from build123d import *

# Parameters (mm, degrees)
BASE_FLANGE1_DEPTH      = 300
CUT_EXTRUDE1_DEPTH      = 303.226736077
CUT_EXTRUDE1_DEPTH_BACK = 303.226736077
SKETCH7_R               = 3


# Sheet-metal steps are written as plain solids
with BuildPart() as part:
    # Sketch2 → Base-Flange1 (new body)
    with BuildSketch(Plane(origin=(0, 0, 0), x_dir=(0, 0, -1), z_dir=(1, 0, 0))):
        with BuildLine():
            Line((0, 0), (18, 0))
            ThreePointArc((18, 0), (19.414213562, -0.585786438), (20, -2))
            Line((20, -2), (20, -19))
            ThreePointArc((20, -19), (20.292893219, -19.707106781), (21, -20))
            Line((21, -20), (30, -20))
            Line((30, -20), (30, -21))
            Line((30, -21), (21, -21))
            ThreePointArc((21, -21), (19.585786438, -20.414213562), (19, -19))
            Line((19, -19), (19, -2))
            ThreePointArc((19, -2), (18.707106781, -1.292893219), (18, -1))
            Line((18, -1), (0, -1))
            Line((0, -1), (0, 0))
        make_face()
    extrude(amount=BASE_FLANGE1_DEPTH)

    # Sketch7 → Cut-Extrude1 (cut, two sides: drawn at the far end of the back side and taken through both)
    with BuildSketch(Plane(origin=(0, 0, 0), x_dir=(1, 0, 0), z_dir=(0, 1, 0)).offset(-CUT_EXTRUDE1_DEPTH_BACK)):
        with Locations(Location((50, 9, 0), (0, 0, 270))):
            Circle(SKETCH7_R)
        with Locations(Location((150, 9, 0), (0, 0, 270))):
            Circle(SKETCH7_R)
    extrude(amount=CUT_EXTRUDE1_DEPTH + CUT_EXTRUDE1_DEPTH_BACK, mode=Mode.SUBTRACT)


solid = part.part
Here's how the part is built. I have some questions about the finished solid (model axes, mm). A direction names the side the tool comes from. Give positions to 0.01 mm unless a question says otherwise; leave off trailing zeros. Write each loop counter-clockwise with the first axis right and the second up, starting at its lowest first coordinate (ties: lowest second). Pieces come first, ordered by that corner, then holes. Notation, with made-up numbers: (63.25, -6) -> (101.25, -6) arc R21 cw to (101.25, 30) -> close; hole circle Ø8 at (-2, 43). An arc over 180 degrees is marked (long way). Use one line per item in the form item = value. Start each with the question number.
1. On a 3-axis mill with a long thin cutter (end or side, diameter ignored), from which of +Z, -Z, +X, -X, +Y, -Y can I reach the whole of each face in a straight line? I mean faces 1 (the face through (0, -8.9, -19.5)), 2 (the face through (148, -1, -5)), 3 (the face through (148, -10, -20)). Say none if no direction works.
2. Will these pins go through, and if not, where does the flat tip stop? pin 1 Ø12 at (x, y) = (94.5, -18) entering from +Z; pin 2 Ø7 at (x, z) = (117.5, -26) entering from +Y; pin 3 Ø2 at (x, y) = (136, -18.5) entering from -Z.
3. Thinking about a two-plate mould opening in X: for faces 4 (the face through (152.53, -0.51, -7.39)), 5 (the face through (52.974, -0.507, -9.391)), 6 (the face through (148, -20, -25)), 7 (the face through (300, -8.9, -19.5)), which applies, +X half, -X half, draft (parallel to the pull), parting line (faces both ways), or undercut?
4. Imagine slicing it at A-A on z = -9. List the corners of the cut face in (x, y) for me.
5. If I drill on L1, parallel to X at y = -0.35, z = -9; L2, parallel to Z at x = 221.5, y = -7.5; L3, parallel to Y at x = 255, z = -22.5, over which ranges is the centre line in solid material (lowest first)?
6. Imagine slicing it at C-C on x = 150. List the corners of the cut face in (y, z) for me.
7. Imagine slicing it at B-B on x = 202. List the corners of the cut face in (y, z) for me, plus the area to 3 significant figures.
Entries:
q1.face_1 = +Z, -Z, -X, +Y, -Y
q1.face_2 = +Z, +X, -X, -Y
q1.face_3 = -Z, +X, -X, +Y
q2.pin_1 = -19
q2.pin_2 = -20
q2.pin_3 = -20.13
q3.face_4 = undercut
q3.face_5 = undercut
q3.face_6 = draft
q3.face_7 = +X half
q4.outline = (0, -1) -> (47, -1) -> (47, 0) -> (0, 0) -> close; (53, -1) -> (147, -1) -> (147, 0) -> (53, 0) -> close; (153, -1) -> (300, -1) -> (300, 0) -> (153, 0) -> close
q5.L1 = 0 to 47, 53 to 147, 153 to 300
q5.L2 = -20 to -19
q5.L3 = -21 to -20
q6.outline = (-21, -30) -> (-20, -30) -> (-20, -21) arc R1 cw to (-19, -20) -> (-2, -20) arc R2 ccw to (0, -18) -> (0, -12) -> (-1, -12) -> (-1, -18) arc R1 cw to (-2, -19) -> (-19, -19) arc R2 ccw to (-21, -21) -> close; (-1, -6) -> (0, -6) -> (0, 0) -> (-1, 0) -> close
q7.outline = (-21, -30) -> (-20, -30) -> (-20, -21) arc R1 cw to (-19, -20) -> (-2, -20) arc R2 ccw to (0, -18) -> (0, 0) -> (-1, 0) -> (-1, -18) arc R1 cw to (-2, -19) -> (-19, -19) arc R2 ccw to (-21, -21) -> close
q7.area = 48.7 mm²
